from build123d import *

# Parameters (mm, degrees)
SKETCH3_R               = 9.5885
BOSS_EXTRUDE1_DEPTH     = 12.7
SKETCH4_R               = 3.614257139
CUT_EXTRUDE1_DEPTH      = 6.35
CUT_EXTRUDE2_START      = -12.7
CUT_EXTRUDE2_OUTLINE_R  = 3
CUT_EXTRUDE2_DEPTH      = 25.4
CUT_EXTRUDE3_DEPTH      = 126.664030474
CUT_EXTRUDE3_DEPTH_BACK = 126.664030474
SKETCH8_W               = 15.24
SKETCH8_H               = 5.08


# Read off the part's stored shape, not the designer's step: Cut-Extrude2
with BuildPart() as part:
    # Sketch3 → Boss-Extrude1 (new body)
    with BuildSketch(Plane.XY):
        with BuildLine():
            Line((50.652428891, 3.175), (-50.652428891, 3.175))
            Line((-50.652428891, 3.175), (-50.652428891, -3.175))
            Line((-50.652428891, -3.175), (-17.78, -3.175))
            ThreePointArc((-17.78, -3.175), (-14.187897552, -4.662897552), (-12.7, -8.255))
            Line((-12.7, -8.255), (-12.7, -29.595434395))
            ThreePointArc((-12.7, -29.595434395), (-12.814872576, -30.66963627), (-13.154295145, -31.69525691))
            Line((-13.154295145, -31.69525691), (-50.652428891, -114.3))
            Line((-50.652428891, -114.3), (-31.75, -114.3))
            Line((-31.75, -114.3), (-31.75, -109.5375))
            Line((-31.75, -109.5375), (31.75, -109.5375))
            Line((31.75, -109.5375), (31.75, -114.3))
            Line((31.75, -114.3), (50.652428891, -114.3))
            Line((50.652428891, -114.3), (13.154295145, -31.69525691))
            ThreePointArc((13.154295145, -31.69525691), (12.814872576, -30.66963627), (12.7, -29.595434395))
            Line((12.7, -29.595434395), (12.7, -8.255))
            ThreePointArc((12.7, -8.255), (14.187897552, -4.662897552), (17.78, -3.175))
            Line((17.78, -3.175), (50.652428891, -3.175))
            Line((50.652428891, -3.175), (50.652428891, 3.175))
        make_face()
        with Locations((0, -15.875)):
            Circle(SKETCH3_R, mode=Mode.SUBTRACT)
        with BuildLine():
            Line((-7.97501727, -32.575611881), (-37.490421301, -97.595177486))
            ThreePointArc((-37.490421301, -97.595177486), (-37.135167146, -102.446299841), (-32.864716446, -104.775))
            Line((-32.864716446, -104.775), (0, -104.775))
            Line((0, -104.775), (32.864716446, -104.775))
            ThreePointArc((32.864716446, -104.775), (37.135167146, -102.446299841), (37.490421301, -97.595177486))
            Line((37.490421301, -97.595177486), (7.97501727, -32.575611881))
            ThreePointArc((7.97501727, -32.575611881), (6.100612256, -30.404983695), (3.349312415, -29.595434395))
            Line((3.349312415, -29.595434395), (-3.349312415, -29.595434395))
            ThreePointArc((-3.349312415, -29.595434395), (-6.100612256, -30.404983695), (-7.97501727, -32.575611881))
        make_face(mode=Mode.SUBTRACT)
    extrude(amount=BOSS_EXTRUDE1_DEPTH)

    # Sketch4 → Cut-Extrude1 (cut)
    with BuildSketch(Plane(origin=(0, 3.175, 0), x_dir=(1, 0, 0), z_dir=(0, 1, 0))):
        with Locations(Location((-38.1, -6.35, 0), (0, 0, 180))):
            Circle(SKETCH4_R)
        with Locations(Location((38.1, -6.35, 0), (0, 0, 180))):
            Circle(SKETCH4_R)
    extrude(amount=-CUT_EXTRUDE1_DEPTH, mode=Mode.SUBTRACT)

    # Cut-Extrude2 outline → Cut-Extrude2 (cut)
    with BuildSketch(Plane.YZ.offset(CUT_EXTRUDE2_START)):
        with Locations((-15.883331584, 6.35)):
            Circle(CUT_EXTRUDE2_OUTLINE_R)
    extrude(amount=CUT_EXTRUDE2_DEPTH, mode=Mode.SUBTRACT)

    # Sketch8 → Cut-Extrude3 (cut, two sides: drawn at the far end of the back side and taken through both)
    with BuildSketch(Plane.XY.offset(12.7).offset(-CUT_EXTRUDE3_DEPTH_BACK)):
        with Locations((-27.94, -105.41)):
            Rectangle(SKETCH8_W, SKETCH8_H)
        with Locations((27.94, -105.41)):
            Rectangle(SKETCH8_W, SKETCH8_H)
    extrude(amount=CUT_EXTRUDE3_DEPTH + CUT_EXTRUDE3_DEPTH_BACK, mode=Mode.SUBTRACT)


solid = part.part
The model under review builds one solid part; all positions refer to its coordinate system, in mm. A direction names the side the tool comes from. Coordinates: 2 decimals unless noted, no trailing zeros. Loops run counter-clockwise (first coordinate to the right, second up) from the corner with the lowest first, then second, coordinate; pieces in that order, holes last.
(1) Consider section A-A, the plane x = 0. Give the boundary of the cut face in (y, z) (1 decimal), plus the area to 3 significant figures.
Determined:
outline: (-109.5, 0) - (-104.8, 0) - (-104.8, 12.7) - (-109.5, 12.7) - close; (-29.6, 0) - (-25.5, 0) - (-25.5, 12.7) - (-29.6, 12.7) - close; (-6.3, 0) - (3.2, 0) - (3.2, 12.7) - (-6.3, 12.7) - close
area: 233 mm2
(2) Wall thickness on L1, parallel to Y at x = 18, z = 9 (1 decimal); L2, parallel to Z at x = 38, y = 0; L3, parallel to Y at x = 14.5, z = 10.25 (1 decimal): over which ranges is each line inside the solid? List them lowest first.
Determined:
L1: y = -109.5 to -104.8, -54.7 to -42.4, -3.2 to 3.2
L2: z = 0 to 2.74, 9.96 to 12.7
L3: y = -109.5 to -104.8, -46.9 to -34.7, -4.4 to 3.2
(3) Insertion check: P1, Ø3.5, axis at y = -15.88, z = 6.35, coming from the +X side; P2, Ø3.5, axis at x = 1, z = 9.5, coming from the -Y side; P3, Ø2, axis at y = -106, z = 7.5, coming from the -X side; P4, Ø2, axis at y = -105.5, z = 4, coming from the +X side. Each pin has a flat end and moves straight along its axis. Give the tip position at first contact, or say it passes through.
Determined:
P1: passes through
P2: stops at y = -109.54
P3: stops at x = -47.34
P4: stops at x = 47.11
(4) Draft analysis for pull direction X (two halves, no side actions). For faces 1 (the flat face through (1, 3.175, 6)), 2 (the flat face through (-20.32, -106, 6)), 3 (the cylindrical face through (14.15, -4.7, 6.26)), 4 (the flat face through (28, -107.95, 6)), state which applies: +X half, -X half, draft (parallel to the pull), parting line (faces both ways), or undercut.
Determined:
face 1: draft
face 2: undercut
face 3: +X half
face 4: undercut
(5) Consider section C-C, the plane z = 8. Give the number of separate pieces and of enclosed holes in the cut face, plus the area to 3 significant figures.
Determined:
separate pieces: 4
enclosed holes: 1
area: 2,320 mm2
(6) Tool access review of faces 5 (the flat face through (-34, -3.175, 6)), 6 (the flat face through (34, -3.175, 6)), 7 (the cylindrical face through (10.877, -13.112, 5.201)), 8 (the flat face through (0, -109.538, 6)), 9 (the flat face through (-35.56, -106, 6)): name each direction out of +Z, -Z, +X, -X, +Y, -Y from which nothing blocks a thin tool from reaching the whole face with its end or side.
Determined:
face 5: +Z, -Z, -X
face 6: +Z, -Z, +X
face 7: +X, -X
face 8: +Z, -Z, -Y
face 9: +Z, -Z
(7) Consider section B-B, the plane y = -23.5. Give the boundary of the cut face in (x, z).
Determined:
outline: (-12.7, 0) - (-5.81, 0) - (-5.81, 12.7) - (-12.7, 12.7) - close; (5.81, 0) - (12.7, 0) - (12.7, 12.7) - (5.81, 12.7) - close
